from build123d import *

# Parameters (mm, degrees)
ESQUISSE1_R             = 6
EXTRUSION1_DEPTH        = 32
ESQUISSE2_R             = 3.4
ENL_V_MAT_EXTRU_1_DEPTH = 2
CHANFREIN1_SIZE         = 1
ESQUISSE3_R             = 0.5
EXTRUSION2_DEPTH        = 3
EXTRUSION3_DEPTH        = 0.05


with BuildPart() as part:
    # Esquisse1 → Extrusion1 (new body)
    with BuildSketch(Plane(origin=(0, 0, 0), x_dir=(0, 0, -1), z_dir=(1, 0, 0))):
        Circle(ESQUISSE1_R)
    extrude(amount=EXTRUSION1_DEPTH)

    # Esquisse2 → Enlèv. mat.-Extru.1 (cut)
    with BuildSketch(Plane.ZY):
        Circle(ESQUISSE2_R)
    extrude(amount=-ENL_V_MAT_EXTRU_1_DEPTH, mode=Mode.SUBTRACT)

    # Chanfrein1
    chanfrein1_edges = [part.edges().sort_by_distance(p)[0] for p in [
        (32, 0, 6),
    ]]
    chamfer(chanfrein1_edges, length=CHANFREIN1_SIZE)

    # Esquisse3 → Extrusion2 (add)
    with BuildSketch(Plane(origin=(32, 0, 0), x_dir=(0, 0, -1), z_dir=(1, 0, 0))):
        with Locations((0, 0.75)):
            Circle(ESQUISSE3_R)
        with Locations(Location((0, -0.75, 0), (0, 0, 180))):
            Circle(ESQUISSE3_R)
    extrude(amount=EXTRUSION2_DEPTH)

    # Esquisse4 → Extrusion3 (add, symmetric)
    with BuildSketch(Plane.XY):
        Polygon((2, 2.75), (2, -2.75), (-498, -46.494331763), (-498, 46.494331763), align=None)
    extrude(amount=EXTRUSION3_DEPTH, both=True)


solid = part.part
Model file for the job. Use its own axes, mm. Give positions to 0.01 mm unless a question says otherwise; leave off trailing zeros. Order: outer loops, then holes, each group sorted by start corner. A loop starts at its lowest first (then second) coordinate and runs counter-clockwise, first axis right, second up. Notation, with made-up numbers: (8.5, 20) - (24.5, 20) arc R19 cw to (24.5, 46) - close; hole circle Ø3 at (-34.5, 7.5). An arc over 180 degrees is marked (long way). Write item = value, one per line. Start each with the question number.
1. Drop flat-ended pins along their axis: P1, Ø6, axis at x = -366.5, z = -2, coming from the +Y side; P2, Ø6, axis at x = -332.5, z = -2, coming from the +Y side; P3, Ø1, axis at x = -196.5, y = 9, coming from the +Z side; P4, Ø3.5, axis at y = 0, z = -1.5, coming from the -X side. Give the stop position or say it passes through.
2. Probe line 1 along Y through (x, z) = (0.9, 0). List the from-to ranges inside material, lowest first.
3. Cut at A-A, the plane x = -243.5. List the corners of the cut face in (y, z), and give its area (3 significant figures).
4. Cut at B-B, the plane y = -35. List the corners of the cut face in (x, z).
Taken from the geometry:
q1.P1 = 35.19
q1.P2 = 32.21
q1.P3 = 0.05
q1.P4 = -498
q2.line_1 = -6 to -3.4, -2.85 to 2.85, 3.4 to 6
q3.outline = (-24.23, -0.05) - (24.23, -0.05) - (24.23, 0.05) - (-24.23, 0.05) - close
q3.area = 4.85 mm²
q4.outline = (-498, -0.05) - (-366.62, -0.05) - (-366.62, 0.05) - (-498, 0.05) - close
